Verification items for this drawing (mm, ordinates from the low corner). Coordinates: 2 decimals unless noted, no trailing zeros. Write each loop counter-clockwise with the first axis right and the second up, starting at its lowest first coordinate (ties: lowest second). Pieces come first, ordered by that corner, then holes. Notation, with made-up numbers: M 70.5,-9.5 L 110.5,-9.5 A11 cw 110.5,-5.5 Z; hole C -25,-29.5 d7. An arc over 180 degrees is marked long. Answer as CSV lines item,"result". Start each with the question number.
1) Section check C-C (y = 0.4). Record the cut outline in (x, z), and give its area (3 significant figures).
2) Section check B-B (z = 6.5). Record the cut outline in (x, y), and give its area (3 significant figures).
3) Section check A-A (x = 6.5). Record the cut outline in (y, z), and give its area (3 significant figures).
4) Draft check along Y on the marked faces 1, 2, 3 and 4. Enter one of: +Y half, -Y half, draft (parallel to the pull), parting line (faces both ways), or undercut.
5) Section check D-D (y = 5). Record the cut outline in (x, z).
6) Material ranges on L1, parallel to Z at x = 6.5, y = 5.6; L2, parallel to Y at x = 5.75, z = 12.25; L3, parallel to X at y = 2, z = 6.75, recorded low to high. Write a range as [from, to].
7) Go/stop test with flat-tipped pins: pin 1 Ø1.5 at (y, z) = (1.5, 9.5) entering from -X; pin 2 Ø1.5 at (x, y) = (8.5, 4) entering from -Z. Record where each tip stops, or that it passes through.
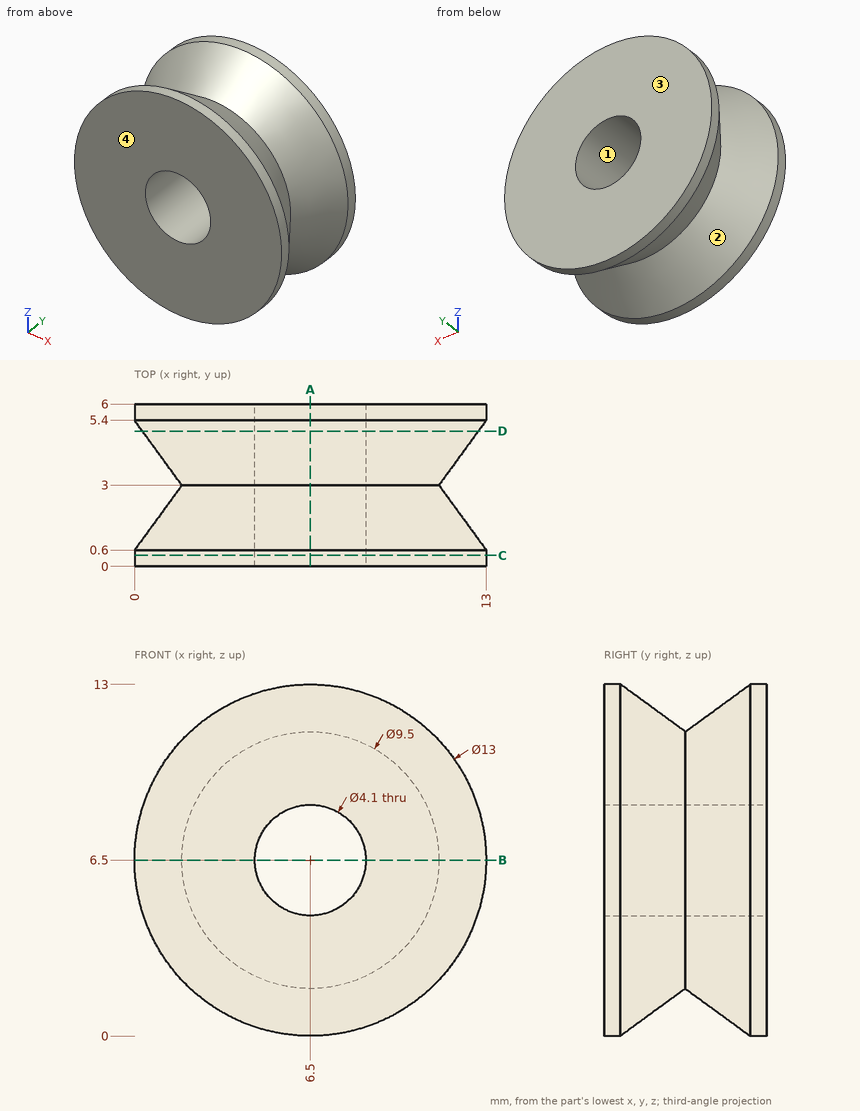
Results found:
1,outline,"C 6.5,6.5 d13; hole C 6.5,6.5 d4.1"
1,area,"120 mm2"
2,outline,"M 0,0 L 4.45,0 L 4.45,6 L 0,6 L 0,5.4 L 1.75,3 L 0,0.6 Z; M 8.55,0 L 13,0 L 13,0.6 L 11.25,3 L 13,5.4 L 13,6 L 8.55,6 Z"
2,area,"45.0 mm2"
3,outline,"M 0,0 L 0.6,0 L 3,1.75 L 5.4,0 L 6,0 L 6,4.45 L 0,4.45 Z; M 0,8.55 L 6,8.55 L 6,13 L 5.4,13 L 3,11.25 L 0.6,13 L 0,13 Z"
3,area,"45.0 mm2"
4,face 1,"draft"
4,face 2,"undercut"
4,face 3,"+Y half"
4,face 4,"-Y half"
5,outline,"C 6.5,6.5 d12.42; hole C 6.5,6.5 d4.1"
6,L1,"z = [0, 4.45], [8.55, 13]"
6,L2,"y = [0, 1.56], [4.44, 6]"
6,L3,"x = [1.03, 4.47], [8.53, 11.97]"
7,pin 1,"stops at x = 0.75"
7,pin 2,"stops at z = 0.77"
